Source: CAD feature listing. Evaluate the final solid. Frame: model axes, mm. A direction names the side the tool comes from. Give positions to 0.01 mm unless a question says otherwise; leave off trailing zeros. Loops run counter-clockwise (first coordinate to the right, second up) from the corner with the lowest first, then second, coordinate; pieces in that order, holes last. Notation, with made-up numbers: (-7, -10.5) -> (13, -10.5) arc R23 ccw to (13, 7.5) -> close; hole circle Ø9 at (70.25, 49.25). An arc over 180 degrees is marked (long way). Return JSON: item names as keys, results as strings. Group by question number.
(1) Ray query, line 1 (X direction, y = -10, z = -30); line 2 (Y direction, x = -28.7, z = -20); line 3 (Z direction, x = -13, y = 6). Return the intervals inside material, ascending. Write a range as from..to.
(2) Cut plane C-C on x = -18. Return loops of the section in (y, z), then the cut area to 3 significant figures.
(3) Pin query (flat end, axial travel): pin 1 (0.6 mm diameter, centred on y = -3.5, z = -39, fed in from -X); pin 2 (8 mm diameter, centred on y = 0, z = -20, fed in from -X); pin 3 (1.6 mm diameter, centred on y = -0.5, z = -38.5, fed in from +X). Return the tip coordinate at first contact, or that it passes through.
(4) Access query for faces 1 (the face through (-17, 0, -39)), 2 (the face through (-30, -6, -20)), 3 (the face through (21, 0, -38)). Directions: +Z, -Z, +X, -X, +Y, -Y. A direction counts if a zero-diameter tool reaches every point of the face in a straight line with its end or side. Return the directions, or none.
(5) Draft query along Z for faces 4 (the face through (0, 0, -2)), 5 (the face through (0, 0, 0)), 6 (the face through (-28.717, -0.35, -38.647)). Return one class per face: released by +Z, released by -Z, zero draft, split by the parting line, or undercut.
(6) Cut plane A-A on y = 0. Return loops of the section in (x, z), then the cut area to 3 significant figures.
(7) Cut plane B-B on z = -20. Return loops of the section in (x, y), then the cut area to 3 significant figures.
(8) Cut plane D-D on z = -28.5. Return loops of the section in (x, y).
```python
from build123d import *

# Parameters (mm, degrees)
SKETCH1_W                      = 60
SKETCH1_H                      = 50
BASE_FLANGE1_DEPTH             = 2
EDGE_FLANGE1_STRIP_W           = 13
EDGE_FLANGE1_STRIP_H           = 2
EDGE_FLANGE1_STRIP_CUT_DEPTH   = 50
EDGE_FLANGE1_STRIP_2_W         = 13
EDGE_FLANGE1_STRIP_2_H         = 2
EDGE_FLANGE1_STRIP_CUT_2_DEPTH = 50
EDGE_FLANGE1_DEPTH             = 50
EDGE_FLANGE1_BEND_DEPTH        = 50
EDGE_FLANGE2_STRIP_W           = 13
EDGE_FLANGE2_STRIP_H           = 2
EDGE_FLANGE2_STRIP_CUT_DEPTH   = 50
EDGE_FLANGE2_STRIP_2_W         = 13
EDGE_FLANGE2_STRIP_2_H         = 2
EDGE_FLANGE2_STRIP_CUT_2_DEPTH = 50
EDGE_FLANGE2_DEPTH             = 50
EDGE_FLANGE2_BEND_DEPTH        = 50
SKETCH20_R                     = 5
CUT_EXTRUDE2_DEPTH             = 77.321687612


# Sheet-metal steps are written as plain solids
with BuildPart() as part:
    # Sketch1 → Base-Flange1 (new body)
    with BuildSketch(Plane.XY):
        Rectangle(SKETCH1_W, SKETCH1_H)
    extrude(amount=-BASE_FLANGE1_DEPTH)

    # Edge-Flange1 strip (across the edge) → Edge-Flange1 strip cut (cut)
    with BuildSketch(Plane(origin=(30, 25, -2), x_dir=(-1, 0, 0), z_dir=(0, -1, 0))):
        with Locations((-2, -1)):
            Rectangle(EDGE_FLANGE1_STRIP_W, EDGE_FLANGE1_STRIP_H)
    extrude(amount=EDGE_FLANGE1_STRIP_CUT_DEPTH, mode=Mode.SUBTRACT)

    # Edge-Flange1 strip 2 (across the edge) → Edge-Flange1 strip cut 2 (cut)
    with BuildSketch(Plane(origin=(-30, -25, -2), x_dir=(1, 0, 0), z_dir=(0, 1, 0))):
        with Locations((-2, -1)):
            Rectangle(EDGE_FLANGE1_STRIP_2_W, EDGE_FLANGE1_STRIP_2_H)
    extrude(amount=EDGE_FLANGE1_STRIP_CUT_2_DEPTH, mode=Mode.SUBTRACT)

    # Edge-Flange1 section (across the edge) → Edge-Flange1 (add)
    with BuildSketch(Plane(origin=(30, 25, -2), x_dir=(-1, 0, 0), z_dir=(0, -1, 0))):
        with BuildLine():
            Line((0, 2.5), (0, 38))
            Line((0, 38), (2, 38))
            Line((2, 38), (2, 2.5))
            ThreePointArc((2, 2.5), (2.732233047, 0.732233047), (4.5, 0))
            Line((4.5, 0), (4.5, -2))
            ThreePointArc((4.5, -2), (1.318019485, -0.681980515), (0, 2.5))
        make_face()
    extrude(amount=EDGE_FLANGE1_DEPTH)

    # Edge-Flange1 section 2 (across the edge) → Edge-Flange1 bend (add)
    with BuildSketch(Plane(origin=(-30, -25, -2), x_dir=(1, 0, 0), z_dir=(0, 1, 0))):
        with BuildLine():
            Line((0, 2.5), (0, 38))
            Line((0, 38), (2, 38))
            Line((2, 38), (2, 2.5))
            ThreePointArc((2, 2.5), (2.732233047, 0.732233047), (4.5, 0))
            Line((4.5, 0), (4.5, -2))
            ThreePointArc((4.5, -2), (1.318019485, -0.681980515), (0, 2.5))
        make_face()
    extrude(amount=EDGE_FLANGE1_BEND_DEPTH)

    # Edge-Flange2 strip (across the edge) → Edge-Flange2 strip cut (cut)
    with BuildSketch(Plane(origin=(28, 25, -40), x_dir=(0, 0, 1), z_dir=(0, -1, 0))):
        with Locations((-2, -1)):
            Rectangle(EDGE_FLANGE2_STRIP_W, EDGE_FLANGE2_STRIP_H)
    extrude(amount=EDGE_FLANGE2_STRIP_CUT_DEPTH, mode=Mode.SUBTRACT)

    # Edge-Flange2 strip 2 (across the edge) → Edge-Flange2 strip cut 2 (cut)
    with BuildSketch(Plane(origin=(-28, -25, -40), x_dir=(0, 0, 1), z_dir=(0, 1, 0))):
        with Locations((-2, -1)):
            Rectangle(EDGE_FLANGE2_STRIP_2_W, EDGE_FLANGE2_STRIP_2_H)
    extrude(amount=EDGE_FLANGE2_STRIP_CUT_2_DEPTH, mode=Mode.SUBTRACT)

    # Edge-Flange2 section (across the edge) → Edge-Flange2 (add)
    with BuildSketch(Plane(origin=(28, 25, -40), x_dir=(0, 0, 1), z_dir=(0, -1, 0))):
        with BuildLine():
            Line((0, 2.5), (0, 11))
            Line((0, 11), (2, 11))
            Line((2, 11), (2, 2.5))
            ThreePointArc((2, 2.5), (2.732233047, 0.732233047), (4.5, 0))
            Line((4.5, 0), (4.5, -2))
            ThreePointArc((4.5, -2), (1.318019485, -0.681980515), (0, 2.5))
        make_face()
    extrude(amount=EDGE_FLANGE2_DEPTH)

    # Edge-Flange2 section 2 (across the edge) → Edge-Flange2 bend (add)
    with BuildSketch(Plane(origin=(-28, -25, -40), x_dir=(0, 0, 1), z_dir=(0, 1, 0))):
        with BuildLine():
            Line((0, 2.5), (0, 11))
            Line((0, 11), (2, 11))
            Line((2, 11), (2, 2.5))
            ThreePointArc((2, 2.5), (2.732233047, 0.732233047), (4.5, 0))
            Line((4.5, 0), (4.5, -2))
            ThreePointArc((4.5, -2), (1.318019485, -0.681980515), (0, 2.5))
        make_face()
    extrude(amount=EDGE_FLANGE2_BEND_DEPTH)

    # Sketch20 → Cut-Extrude2 (cut, through all)
    with BuildSketch(Plane(origin=(30, 0, 0), x_dir=(0, 0, -1), z_dir=(1, 0, 0))):
        with Locations((20, 0)):
            Circle(SKETCH20_R)
    extrude(amount=-CUT_EXTRUDE2_DEPTH, mode=Mode.SUBTRACT)


solid = part.part
```
Answers:
{
 "1": {"line 1": "-30..-28, 28..30", "line 2": "-25..-5, 5..25", "line 3": "-2..0"},
 "2": {"outline": "(-25, -40) -> (25, -40) -> (25, -38) -> (-25, -38) -> close; (-25, -2) -> (25, -2) -> (25, 0) -> (-25, 0) -> close", "area": "200 mm²"},
 "3": {"pin 1": "x = -28.66", "pin 2": "through", "pin 3": "x = 29.43"},
 "4": {"face 1": "-Z, +Y, -Y", "face 2": "+Z, -Z, -X, +Y, -Y", "face 3": "+Y, -Y"},
 "5": {"face 4": "undercut", "face 5": "released by +Z", "face 6": "released by -Z"},
 "6": {"outline": "(-30, -35.5) arc R4.5 ccw to (-25.5, -40) -> (-17, -40) -> (-17, -38) -> (-25.5, -38) arc R2.5 cw to (-28, -35.5) -> (-28, -25) -> (-30, -25) -> close; (-30, -15) -> (-28, -15) -> (-28, -4.5) arc R2.5 cw to (-25.5, -2) -> (25.5, -2) arc R2.5 cw to (28, -4.5) -> (28, -15) -> (30, -15) -> (30, -4.5) arc R4.5 ccw to (25.5, 0) -> (-25.5, 0) arc R4.5 ccw to (-30, -4.5) -> close; (17, -40) -> (25.5, -40) arc R4.5 ccw to (30, -35.5) -> (30, -25) -> (28, -25) -> (28, -35.5) arc R2.5 cw to (25.5, -38) -> (17, -38) -> close", "area": "264 mm²"},
 "7": {"outline": "(-30, -25) -> (-28, -25) -> (-28, -5) -> (-30, -5) -> close; (-30, 5) -> (-28, 5) -> (-28, 25) -> (-30, 25) -> close; (28, -25) -> (30, -25) -> (30, -5) -> (28, -5) -> close; (28, 5) -> (30, 5) -> (30, 25) -> (28, 25) -> close", "area": "160 mm²"},
 "8": {"outline": "(-30, -25) -> (-28, -25) -> (-28, 25) -> (-30, 25) -> close; (28, -25) -> (30, -25) -> (30, 25) -> (28, 25) -> close"}
}
